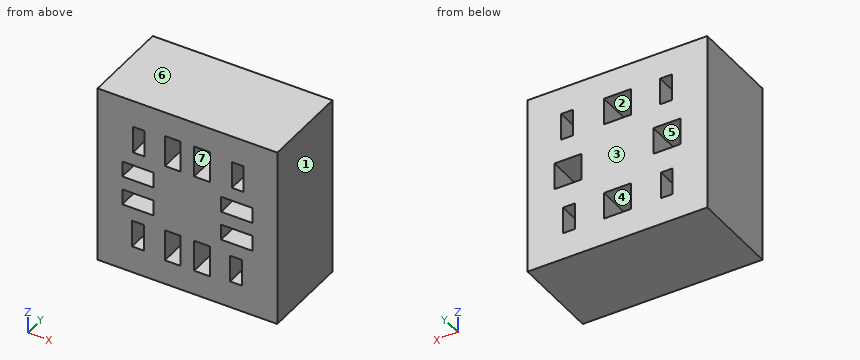
```python
from build123d import *

# Parameters (mm, degrees)
SKETCH_208_W             = 40
SKETCH_208_H             = 40
SKETCH_208_W_2           = 6
SKETCH_208_H_2           = 6
EXTRUDE_1_DEPTH          = 10
SKETCH_1_W               = 40
SKETCH_1_H               = 40
SKETCH_1_W_2             = 3.5
SKETCH_1_H_2             = 7
SKETCH_1_W_3             = 7
SKETCH_1_H_3             = 3.5
EXTRUDE_5_DEPTH          = 10
CUT_EXTRUDE_1_DEPTH      = 31
CUT_EXTRUDE_1_DEPTH_BACK = 31
SKETCH_1_6_W             = 2.6
SKETCH_1_6_H             = 6
CUT_EXTRUDE_2_DEPTH      = 31
CUT_EXTRUDE_2_DEPTH_BACK = 31
SKETCH_1_7_W             = 2.6
SKETCH_1_7_H             = 6
CUT_EXTRUDE_3_DEPTH      = 31
CUT_EXTRUDE_3_DEPTH_BACK = 31
SKETCH_1_8_W             = 2.6
SKETCH_1_8_H             = 6
CUT_EXTRUDE_4_DEPTH      = 31
CUT_EXTRUDE_4_DEPTH_BACK = 31
SKETCH_1_9_W             = 2.6
SKETCH_1_9_H             = 6


with BuildPart() as part:
    # Sketch 208 → Бобышка-Вытянуть1 (new body)
    with BuildSketch(Plane(origin=(0, 0, 0), x_dir=(1, 0, 0), z_dir=(0, 1, 0))):
        Rectangle(SKETCH_208_W, SKETCH_208_H)
        with Locations((11, 0)):
            Rectangle(SKETCH_208_W_2, SKETCH_208_H_2, mode=Mode.SUBTRACT)
        with Locations((-11, 0)):
            Rectangle(SKETCH_208_W_2, SKETCH_208_H_2, mode=Mode.SUBTRACT)
        with Locations((0, -11)):
            Rectangle(SKETCH_208_W_2, SKETCH_208_H_2, mode=Mode.SUBTRACT)
        with Locations((0, 11)):
            Rectangle(SKETCH_208_W_2, SKETCH_208_H_2, mode=Mode.SUBTRACT)
    extrude(amount=EXTRUDE_1_DEPTH)

    # Эскиз1 → Бобышка-Вытянуть5 (add)
    with BuildSketch(Plane.XZ):
        Rectangle(SKETCH_1_W, SKETCH_1_H)
        with Locations((-3.25, -11)):
            Rectangle(SKETCH_1_W_2, SKETCH_1_H_2, mode=Mode.SUBTRACT)
        with Locations((3.25, -11)):
            Rectangle(SKETCH_1_W_2, SKETCH_1_H_2, mode=Mode.SUBTRACT)
        with Locations((-11, -3.25)):
            Rectangle(SKETCH_1_W_3, SKETCH_1_H_3, mode=Mode.SUBTRACT)
        with Locations((-11, 3.25)):
            Rectangle(SKETCH_1_W_3, SKETCH_1_H_3, mode=Mode.SUBTRACT)
        with Locations((11, 3.25)):
            Rectangle(SKETCH_1_W_3, SKETCH_1_H_3, mode=Mode.SUBTRACT)
        with Locations((11, -3.25)):
            Rectangle(SKETCH_1_W_3, SKETCH_1_H_3, mode=Mode.SUBTRACT)
        with Locations((-3.25, 11)):
            Rectangle(SKETCH_1_W_2, SKETCH_1_H_2, mode=Mode.SUBTRACT)
        with Locations((3.25, 11)):
            Rectangle(SKETCH_1_W_2, SKETCH_1_H_2, mode=Mode.SUBTRACT)
    extrude(amount=EXTRUDE_5_DEPTH)

    # Эскиз1<6> → Вырез-Вытянуть1 (cut, two sides: drawn at the far end of the back side and taken through both)
    with BuildSketch(Plane.XZ.offset(-CUT_EXTRUDE_1_DEPTH_BACK)):
        with Locations((-10.806551552, 11)):
            Rectangle(SKETCH_1_6_W, SKETCH_1_6_H)
    extrude(amount=CUT_EXTRUDE_1_DEPTH + CUT_EXTRUDE_1_DEPTH_BACK, mode=Mode.SUBTRACT)

    # Эскиз1<7> → Вырез-Вытянуть2 (cut, two sides: drawn at the far end of the back side and taken through both)
    with BuildSketch(Plane.XZ.offset(-CUT_EXTRUDE_2_DEPTH_BACK)):
        with Locations((11.206646971, 11)):
            Rectangle(SKETCH_1_7_W, SKETCH_1_7_H)
    extrude(amount=CUT_EXTRUDE_2_DEPTH + CUT_EXTRUDE_2_DEPTH_BACK, mode=Mode.SUBTRACT)

    # Эскиз1<8> → Вырез-Вытянуть3 (cut, two sides: drawn at the far end of the back side and taken through both)
    with BuildSketch(Plane.XZ.offset(-CUT_EXTRUDE_3_DEPTH_BACK)):
        with Locations((10.793353029, -11)):
            Rectangle(SKETCH_1_8_W, SKETCH_1_8_H)
    extrude(amount=CUT_EXTRUDE_3_DEPTH + CUT_EXTRUDE_3_DEPTH_BACK, mode=Mode.SUBTRACT)

    # Эскиз1<9> → Вырез-Вытянуть4 (cut, two sides: drawn at the far end of the back side and taken through both)
    with BuildSketch(Plane.XZ.offset(-CUT_EXTRUDE_4_DEPTH_BACK)):
        with Locations((-11, -11)):
            Rectangle(SKETCH_1_9_W, SKETCH_1_9_H)
    extrude(amount=CUT_EXTRUDE_4_DEPTH + CUT_EXTRUDE_4_DEPTH_BACK, mode=Mode.SUBTRACT)


solid = part.part
```
Input: part model. Units: mm. Frame: model coordinates. Face numbers are marked on the shaded views. A direction names the side the tool comes from. Coordinates: 2 decimals unless noted, no trailing zeros. Write each loop counter-clockwise with the first axis right and the second up, starting at its lowest first coordinate (ties: lowest second). Pieces come first, ordered by that corner, then holes.
1) Set-up query: the marked faces 4, 5, 6 and 7. Return all of +Z, -Z, +X, -X, +Y, -Y with unobstructed straight access to the full face (end or side cutting, diameter ignored); none if empty.
2) Mould query, pull axis X, two halves, no side actions, for the marked faces 1, 2 and 3. Classes: pulls with the +X half, pulls with the -X half, needs draft (parallel to the pull), parting line crosses it, or undercut.
3) Section D-D on x = -11.5. Output: boundary loops of the cut face in (y, z).
4) Section B-B on x = 13. Output: boundary loops of the cut face in (y, z).
5) Material intervals for line 1 along Z through (x, y) = (-4, -1); line 2 along X through (y, z) = (5.5, -8.5), sorted ascending.
6) Pin query (flat end, axial travel): pin 1 Ø2.5 at (x, z) = (0, -12.5) entering from +Y. Return the tip coordinate at first contact, or that it passes through.
7) Section C-C on z = 13.5. Output: boundary loops of the cut face in (x, y), and give its area (3 significant figures).
8) Section A-A on z = 2.5. Output: boundary loops of the cut face in (x, y).
Check result:
1. face 4: +Y
1. face 5: +Y, -Y
1. face 6: +Z, +X, -X, +Y, -Y
1. face 7: -Y
2. face 1: pulls with the +X half
2. face 2: undercut
2. face 3: needs draft
3. outline: (-10, -20) - (10, -20) - (10, -14) - (-10, -14) - close; (-10, -8) - (10, -8) - (10, -3) - (0, -3) - (0, -5) - (-10, -5) - close; (-10, -1.5) - (0, -1.5) - (0, 1.5) - (-10, 1.5) - close; (-10, 5) - (0, 5) - (0, 3) - (10, 3) - (10, 8) - (-10, 8) - close; (-10, 14) - (10, 14) - (10, 20) - (-10, 20) - close
4. outline: (-10, -20) - (10, -20) - (10, -3) - (0, -3) - (0, -5) - (-10, -5) - close; (-10, -1.5) - (0, -1.5) - (0, 1.5) - (-10, 1.5) - close; (-10, 5) - (0, 5) - (0, 3) - (10, 3) - (10, 20) - (-10, 20) - close
5. line 1: z = -20 to -14.5, -7.5 to 7.5, 14.5 to 20
5. line 2: x = -20 to -12.3, -9.7 to -3, 3 to 9.49, 12.09 to 20
6. pin 1: stops at y = 0
7. outline: (-20, -10) - (-12.11, -10) - (-12.11, 10) - (-20, 10) - close; (-9.51, -10) - (-5, -10) - (-5, 0) - (-3, 0) - (-3, 10) - (-9.51, 10) - close; (-1.5, -10) - (1.5, -10) - (1.5, 0) - (-1.5, 0) - close; (3, 0) - (5, 0) - (5, -10) - (9.91, -10) - (9.91, 10) - (3, 10) - close; (12.51, -10) - (20, -10) - (20, 10) - (12.51, 10) - close
7. area: 566 mm2
8. outline: (-20, -10) - (-14.5, -10) - (-14.5, 0) - (-14, 0) - (-14, 10) - (-20, 10) - close; (-8, 0) - (-7.5, 0) - (-7.5, -10) - (7.5, -10) - (7.5, 0) - (8, 0) - (8, 10) - (-8, 10) - close; (14, 0) - (14.5, 0) - (14.5, -10) - (20, -10) - (20, 10) - (14, 10) - close
